CAD build for the part. Positions are in the model's coordinates, mm. Face numbers are marked on the shaded views. A direction names the side the tool comes from. Round coordinates to 2 decimals unless told otherwise and drop trailing zeros. Order: outer loops, then holes, each group sorted by start corner. A loop starts at its lowest first (then second) coordinate and runs counter-clockwise, first axis right, second up. Notation, with made-up numbers: (-12, 58.5) -> (17, 58.5) arc R17 ccw to (17, 69.5) -> close; hole circle Ø6 at (48, 38). An arc over 180 degrees is marked (long way). Return JSON: item names as keys, results as strings. Group by question number.
Q1. Which spindle directions (+Z, -Z, +X, -X, +Y, -Y) get a long thin tool onto all of the face, cutting with end or side? Do the marked faces 1 and 2. Say none if no direction does.
Q2. Probe line 1 along X through (y, z) = (8.65, 0); line 2 along Y through (x, z) = (-1, 1); line 3 along Y through (x, z) = (-3.75, -1.75). List the from-to ranges inside material, lowest first.
Q3. Cut at B-B (y = 1.5). Write the cut outline in (x, z).
Q4. Cut at D-D (x = 3.5). Write the cut outline in (y, z).
Q5. Flat gauge pins, fed straight in: pin 1 (2.5 mm diameter, centred on x = 0, z = 0, fed in from +Y); pin 2 (1.4 mm diameter, centred on x = 0, z = 0, fed in from +Y). Where does each tip first touch, or does it go through?
Q6. Cut at C-C (x = 0). Write the cut outline in (y, z) (3 decimals).
Q7. Mould opens along Z. For the marked faces 3, 4 and 5 say: +Z half, -Z half, draft (parallel to the pull), parting line (faces both ways), or undercut.
Q8. Cut at A-A (z = 0). Write the cut outline in (x, y).
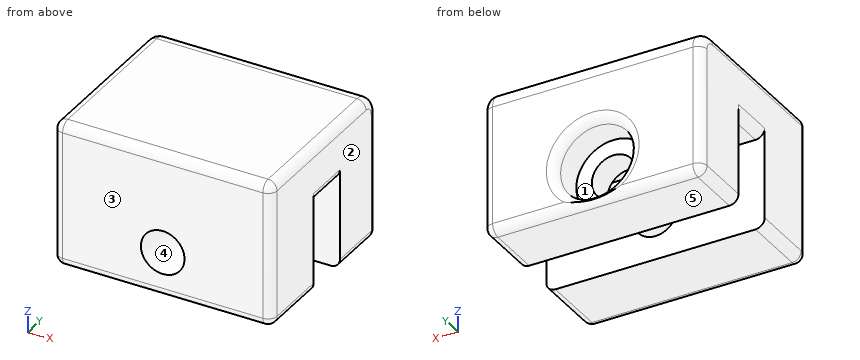
from build123d import *

# Parameters (mm, degrees)
SKETCH1_W               = 12
SKETCH1_H               = 5
BOSS_EXTRUDE1_DEPTH     = 4
SKETCH2_W               = 12
SKETCH2_H               = 6.5
BOSS_EXTRUDE2_DEPTH     = 3
SKETCH3_W               = 12
SKETCH3_H               = 8
BOSS_EXTRUDE3_DEPTH     = 3.5
CUT_EXTRUDE1_DEPTH      = 7
CUT_EXTRUDE1_DEPTH_BACK = 5
SKETCH4_R               = 1.2
SKETCH5_R               = 2.05
CUT_EXTRUDE2_DEPTH      = 2
FILLET3_R               = 0.5
FILLET6_R               = 1
FILLET7_R               = 0.5


with BuildPart() as part:
    # Sketch1 → Boss-Extrude1 (new body)
    with BuildSketch(Plane(origin=(0, 0, 0), x_dir=(1, 0, 0), z_dir=(0, 1, 0))):
        Rectangle(SKETCH1_W, SKETCH1_H)
    extrude(amount=BOSS_EXTRUDE1_DEPTH)

    # Sketch2 → Boss-Extrude2 (add)
    with BuildSketch(Plane.XY.offset(2.5)):
        with Locations((0, 3.25)):
            Rectangle(SKETCH2_W, SKETCH2_H)
    extrude(amount=BOSS_EXTRUDE2_DEPTH)

    # Sketch3 → Boss-Extrude3 (add)
    with BuildSketch(Plane(origin=(0, 6.5, 0), x_dir=(1, 0, 0), z_dir=(0, 1, 0))):
        with Locations((0, -1.5)):
            Rectangle(SKETCH3_W, SKETCH3_H)
    extrude(amount=BOSS_EXTRUDE3_DEPTH)

    # Sketch4 → Cut-Extrude1 (cut, two sides: drawn at the far end of the back side and taken through both)
    with BuildSketch(Plane(origin=(0, 4, 0), x_dir=(1, 0, 0), z_dir=(0, 1, 0)).offset(-CUT_EXTRUDE1_DEPTH_BACK)):
        with Locations(Location((0, 0, 0), (0, 0, 90))):
            Circle(SKETCH4_R)
    extrude(amount=CUT_EXTRUDE1_DEPTH + CUT_EXTRUDE1_DEPTH_BACK, mode=Mode.SUBTRACT)

    # Sketch5 → Cut-Extrude2 (cut)
    with BuildSketch(Plane(origin=(0, 10, 0), x_dir=(1, 0, 0), z_dir=(0, 1, 0))):
        with Locations(Location((0, 0, 0), (0, 0, 270))):
            Circle(SKETCH5_R)
    extrude(amount=-CUT_EXTRUDE2_DEPTH, mode=Mode.SUBTRACT)

    # Fillet3
    fillet3_edges = [part.edges().sort_by_distance(p)[0] for p in [
        (-6, 5.25, 2.5),
        (6, 5.25, 2.5),
        (0, 0, 5.5),
        (-6, 0, 1.5),
        (0, 0, -2.5),
        (6, 0, 1.5),
        (-6, 2, -2.5),
        (6, 2, -2.5),
    ]]
    fillet(fillet3_edges, radius=FILLET3_R)

    # Fillet6
    fillet6_edges = [part.edges().sort_by_distance(p)[0] for p in [
        (0, 10, 5.5),
    ]]
    fillet(fillet6_edges, radius=FILLET6_R)

    # Fillet7
    # the kernel refuses this fillet: 0.5 mm, written as the material it takes off along each edge
    with BuildSketch(Plane(origin=(5.5, 0.5, 5), x_dir=(0, 0, 1), z_dir=(1, 0, 0))) as fillet7_piece_1_section:
        Polygon((0, 0), (FILLET7_R, 0), (FILLET7_R, FILLET7_R), (0, FILLET7_R), align=None)
    fillet7_piece_1 = extrude(amount=FILLET7_R, mode=Mode.PRIVATE)
    fillet7_piece_1 = fillet7_piece_1 - Plane(origin=(5.5, 0.5, 5), x_dir=(0, 0.7071067811865475, -0.7071067811865475), z_dir=(1, 0, 0)) * Sphere(FILLET7_R, mode=Mode.PRIVATE)
    add(fillet7_piece_1, mode=Mode.SUBTRACT)
    with BuildSketch(Plane(origin=(-5.5, 0.5, 5), x_dir=(-1, 0, 0), z_dir=(0, 0, 1))) as fillet7_piece_2_section:
        Polygon((0, 0), (FILLET7_R, 0), (FILLET7_R, FILLET7_R), (0, FILLET7_R), align=None)
    fillet7_piece_2 = extrude(amount=FILLET7_R, mode=Mode.PRIVATE)
    fillet7_piece_2 = fillet7_piece_2 - Plane(origin=(-5.5, 0.5, 5), x_dir=(0.7071067811865475, 0.7071067811865475, 0), z_dir=(0, 0, 1)) * Sphere(FILLET7_R, mode=Mode.PRIVATE)
    add(fillet7_piece_2, mode=Mode.SUBTRACT)
    with BuildSketch(Plane(origin=(5.5, 9.5, -2), x_dir=(0, 1, 0), z_dir=(1, 0, 0))) as fillet7_piece_3_section:
        Polygon((0, 0), (FILLET7_R, 0), (FILLET7_R, -FILLET7_R), (0, -FILLET7_R), align=None)
    fillet7_piece_3 = extrude(amount=FILLET7_R, mode=Mode.PRIVATE)
    fillet7_piece_3 = fillet7_piece_3 - Plane(origin=(5.5, 9.5, -2), x_dir=(0, -0.7071067811865475, 0.7071067811865475), z_dir=(1, 0, 0)) * Sphere(FILLET7_R, mode=Mode.PRIVATE)
    add(fillet7_piece_3, mode=Mode.SUBTRACT)
    with BuildSketch(Plane(origin=(-5.5, 9.5, -2), x_dir=(0, 1, 0), z_dir=(-1, 0, 0))) as fillet7_piece_4_section:
        Polygon((0, 0), (FILLET7_R, 0), (FILLET7_R, FILLET7_R), (0, FILLET7_R), align=None)
    fillet7_piece_4 = extrude(amount=FILLET7_R, mode=Mode.PRIVATE)
    fillet7_piece_4 = fillet7_piece_4 - Plane(origin=(-5.5, 9.5, -2), x_dir=(0, -0.7071067811865475, 0.7071067811865475), z_dir=(-1, 0, 0)) * Sphere(FILLET7_R, mode=Mode.PRIVATE)
    add(fillet7_piece_4, mode=Mode.SUBTRACT)
    with BuildSketch(Plane(origin=(6, 10, 4.5), x_dir=(0, -1, 0), z_dir=(0, 0, -1))) as fillet7_piece_5:
        with BuildLine():
            CenterArc((FILLET7_R, FILLET7_R), FILLET7_R, 180, 90)
            Line((0, FILLET7_R), (0, 0))
            Line((0, 0), (FILLET7_R, 0))
        make_face()
    extrude(amount=6.5, mode=Mode.SUBTRACT)
    with BuildSketch(Plane(origin=(6, 9, 4.5), x_dir=(0, 1, 0), z_dir=(0, 0, -1))) as fillet7_piece_6:
        with BuildLine():
            CenterArc((1 - FILLET7_R, -FILLET7_R), FILLET7_R, 0, 90)
            Line((1, -FILLET7_R), (1, 0))
            Line((1, 0), (1 - FILLET7_R, 0))
        make_face()
    revolve(axis=Axis((6, 9, 4.5), (1, 0, 0)), revolution_arc=90, mode=Mode.SUBTRACT)
    with BuildSketch(Plane(origin=(-6, 9, 5.5), x_dir=(1, 0, 0), z_dir=(0, -1, 0)), Plane(origin=(6, 9, 5.5), x_dir=(0, 0, -1), z_dir=(0, -1, 0))) as fillet7_piece_7:
        with BuildLine():
            CenterArc((FILLET7_R, -FILLET7_R), FILLET7_R, 90, 90)
            Line((0, -FILLET7_R), (0, 0))
            Line((0, 0), (FILLET7_R, 0))
        make_face()
    extrude(amount=8.5, mode=Mode.SUBTRACT)
    with BuildSketch(Plane(origin=(-6, 9, 4.5), x_dir=(0, 1, 0), z_dir=(0, 0, -1))) as fillet7_piece_8:
        with BuildLine():
            CenterArc((1 - FILLET7_R, FILLET7_R), FILLET7_R, 270, 90)
            Line((1 - FILLET7_R, 0), (1, 0))
            Line((1, 0), (1, FILLET7_R))
        make_face()
    revolve(axis=Axis((-6, 9, 4.5), (1, 0, 0)), revolution_arc=90, mode=Mode.SUBTRACT)
    with BuildSketch(Plane(origin=(-6, 5.25, -2.5), x_dir=(1, 0, 0), z_dir=(0, 1, 0)), Plane(origin=(6, 5.25, -2.5), x_dir=(0, 0, 1), z_dir=(0, 1, 0))) as fillet7_piece_9:
        with BuildLine():
            CenterArc((FILLET7_R, -FILLET7_R), FILLET7_R, 90, 90)
            Line((0, -FILLET7_R), (0, 0))
            Line((0, 0), (FILLET7_R, 0))
        make_face()
    extrude(amount=4.25, mode=Mode.SUBTRACT)
    with BuildSketch(Plane(origin=(-6, 10, -2), x_dir=(1, 0, 0), z_dir=(0, 0, 1))) as fillet7_piece_10:
        with BuildLine():
            CenterArc((FILLET7_R, -FILLET7_R), FILLET7_R, 90, 90)
            Line((0, -FILLET7_R), (0, 0))
            Line((0, 0), (FILLET7_R, 0))
        make_face()
    extrude(amount=6.5, mode=Mode.SUBTRACT)
    with BuildSketch(Plane(origin=(5.5, 10, -2.5), x_dir=(0, 0, 1), z_dir=(-1, 0, 0))) as fillet7_piece_11:
        with BuildLine():
            CenterArc((FILLET7_R, -FILLET7_R), FILLET7_R, 90, 90)
            Line((0, -FILLET7_R), (0, 0))
            Line((0, 0), (FILLET7_R, 0))
        make_face()
    extrude(amount=11, mode=Mode.SUBTRACT)
    with BuildSketch(Plane(origin=(0, 10, 0), x_dir=(0, 0, 1), z_dir=(-1, 0, 0))) as fillet7_piece_12:
        with BuildLine():
            CenterArc((2.05 + FILLET7_R, -FILLET7_R), FILLET7_R, 90, 90)
            Line((2.05, -FILLET7_R), (2.05, 0))
            Line((2.05, 0), (2.05 + FILLET7_R, 0))
        make_face()
    revolve(axis=Axis((0, 10, 0), (0, 1, 0)), mode=Mode.SUBTRACT)


solid = part.part
Solution:
{
 "1": {"face 1": "+Y", "face 2": "+Z, -Z, +X, +Y, -Y"},
 "2": {"line 1": "x = -6 to -2.05, 2.05 to 6", "line 2": "y = 0 to 4, 6.5 to 8", "line 3": "y = 0 to 4, 6.5 to 10"},
 "3": {"outline": "(-6, -2) arc R0.5 ccw to (-5.5, -2.5) -> (5.5, -2.5) arc R0.5 ccw to (6, -2) -> (6, 5) arc R0.5 ccw to (5.5, 5.5) -> (-5.5, 5.5) arc R0.5 ccw to (-6, 5) -> close; hole circle Ø2.4 at (0, 0)"},
 "4": {"outline": "(0, -2) arc R0.5 ccw to (0.5, -2.5) -> (4, -2.5) -> (4, 2.5) -> (6.5, 2.5) -> (6.5, -2.5) -> (9.5, -2.5) arc R0.5 ccw to (10, -2) -> (10, 4.5) arc R1 ccw to (9, 5.5) -> (0.5, 5.5) arc R0.5 ccw to (0, 5) -> close"},
 "5": {"pin 1": "stops at y = 8", "pin 2": "passes through"},
 "6": {"outline": "(0, -2) arc R0.5 ccw to (0.5, -2.5) -> (4, -2.5) -> (4, -1.2) -> (0, -1.2) -> close; (0, 1.2) -> (4, 1.2) -> (4, 2.5) -> (6.5, 2.5) -> (6.5, 1.2) -> (8, 1.2) -> (8, 2.05) -> (9.5, 2.05) arc R0.5 ccw to (10, 2.55) -> (10, 4.5) arc R1 ccw to (9, 5.5) -> (0.5, 5.5) arc R0.5 ccw to (0, 5) -> close; (6.5, -2.5) -> (9.5, -2.5) arc R0.5 ccw to (9.918, -2.275) arc R0.5 ccw to (9.5, -2.05) -> (8, -2.05) -> (8, -1.2) -> (6.5, -1.2) -> close"},
 "7": {"face 3": "draft", "face 4": "undercut", "face 5": "-Z half"},
 "8": {"outline": "(-6, 0.5) arc R0.5 ccw to (-5.5, 0) -> (-1.2, 0) -> (-1.2, 4) -> (-6, 4) -> close; (-6, 6.5) -> (-1.2, 6.5) -> (-1.2, 8) -> (-2.05, 8) -> (-2.05, 9.5) arc R0.5 ccw to (-2.55, 10) -> (-5.5, 10) arc R0.5 ccw to (-6, 9.5) -> close; (1.2, 0) -> (5.5, 0) arc R0.5 ccw to (6, 0.5) -> (6, 4) -> (1.2, 4) -> close; (1.2, 6.5) -> (6, 6.5) -> (6, 9.5) arc R0.5 ccw to (5.5, 10) -> (2.55, 10) arc R0.5 ccw to (2.05, 9.5) -> (2.05, 8) -> (1.2, 8) -> close"}
}
